```python
from build123d import *

# Parameters (mm, degrees)
SALIENTE_EXTRUIR1_DEPTH = 20
CORTAR_EXTRUIR1_START   = -6.736039
CROQUIS2_W              = 14
CROQUIS2_H              = 7.5
CORTAR_EXTRUIR1_DEPTH   = 6.736039
CORTAR_EXTRUIR2_REACH   = 29.226
CROQUIS3_R              = 1.7
CROQUIS5_W              = 14
CROQUIS5_H              = 5.763961031
CORTAR_EXTRUIR4_DEPTH   = 10
CORTAR_EXTRUIR3_REACH   = 30.507
CROQUIS4_R              = 3.75
CROQUIS4_W              = 5
CROQUIS4_H              = 5
REDONDEO1_R             = 5
REDONDEO2_R             = 5
REDONDEO3_R             = 2


# Some blends are built 0.0001 mm under size
with BuildPart() as part:
    # Croquis1 → Saliente-Extruir1 (new body)
    with BuildSketch(Plane(origin=(0, 0, 0), x_dir=(0, 0, -1), z_dir=(1, 0, 0))):
        Polygon((-3.75, 4.25), (-0.85, 4.25), (3.15, 8.25), (3.15, 16.813961031), (7.65, 16.813961031), (7.65, 6.386038969), (3.75, 2.486038969), (3.75, -4.25), (-3.75, -4.25), align=None)
    extrude(amount=SALIENTE_EXTRUIR1_DEPTH)

    # Croquis2 → Cortar-Extruir1 (cut)
    with BuildSketch(Plane.XZ.offset(4.25).offset(CORTAR_EXTRUIR1_START)):
        with Locations((10, 0)):
            Rectangle(CROQUIS2_W, CROQUIS2_H)
    extrude(amount=CORTAR_EXTRUIR1_DEPTH, mode=Mode.SUBTRACT)

    # Cortar-Extruir2: up to this face of the body (flat: up to its plane)
    cortar_extruir2_end = Plane(part.part.faces().sort_by_distance((20, 4.974035109, -2.43613322))[0])
    # Croquis3 → Cortar-Extruir2 (cut, up to the picked face)
    with BuildSketch(Plane.ZY, mode=Mode.PRIVATE) as cortar_extruir2_sk1:
        Circle(CROQUIS3_R)
    cortar_extruir2_tool1 = split(extrude(cortar_extruir2_sk1.sketch, amount=-CORTAR_EXTRUIR2_REACH, mode=Mode.PRIVATE), bisect_by=cortar_extruir2_end, keep=Keep.BOTH, mode=Mode.PRIVATE)
    add(cortar_extruir2_tool1.solids().sort_by(Axis((0, 0, 0), (1, 0, 0)))[0], mode=Mode.SUBTRACT)

    # Croquis5 → Cortar-Extruir4 (cut)
    with BuildSketch(Plane.XY.offset(-3.15)):
        with Locations((10, 5.368019484)):
            Rectangle(CROQUIS5_W, CROQUIS5_H)
    extrude(amount=CORTAR_EXTRUIR4_DEPTH, mode=Mode.SUBTRACT)

    # Cortar-Extruir3: up to this face of the body (flat: up to its plane)
    cortar_extruir3_end = Plane(part.part.faces().sort_by_distance((10, 10.237705939, -3.15))[0])
    # Croquis4 → Cortar-Extruir3 (cut, up to the picked face)
    with BuildSketch(Plane(origin=(0, 0, -7.65), x_dir=(-1, 0, 0), z_dir=(0, 0, -1)), mode=Mode.PRIVATE) as cortar_extruir3_sk1:
        with Locations((-10, 11.6)):
            Circle(CROQUIS4_R)
    cortar_extruir3_tool1 = split(extrude(cortar_extruir3_sk1.sketch, amount=-CORTAR_EXTRUIR3_REACH, mode=Mode.PRIVATE), bisect_by=cortar_extruir3_end, keep=Keep.BOTH, mode=Mode.PRIVATE)
    # Croquis4 → Cortar-Extruir3 (cut, up to the picked face)
    with BuildSketch(Plane(origin=(0, 0, -7.65), x_dir=(-1, 0, 0), z_dir=(0, 0, -1)), mode=Mode.PRIVATE) as cortar_extruir3_sk2:
        with Locations((-17.5, 14.313961031)):
            Rectangle(CROQUIS4_W, CROQUIS4_H)
    cortar_extruir3_tool2 = split(extrude(cortar_extruir3_sk2.sketch, amount=-CORTAR_EXTRUIR3_REACH, mode=Mode.PRIVATE), bisect_by=cortar_extruir3_end, keep=Keep.BOTH, mode=Mode.PRIVATE)
    # Croquis4 → Cortar-Extruir3 (cut, up to the picked face)
    with BuildSketch(Plane(origin=(0, 0, -7.65), x_dir=(-1, 0, 0), z_dir=(0, 0, -1)), mode=Mode.PRIVATE) as cortar_extruir3_sk3:
        with Locations((-2.5, 14.313961031)):
            Rectangle(CROQUIS4_W, CROQUIS4_H)
    cortar_extruir3_tool3 = split(extrude(cortar_extruir3_sk3.sketch, amount=-CORTAR_EXTRUIR3_REACH, mode=Mode.PRIVATE), bisect_by=cortar_extruir3_end, keep=Keep.BOTH, mode=Mode.PRIVATE)
    # Croquis4 → Cortar-Extruir3 (cut, up to the picked face)
    with BuildSketch(Plane(origin=(0, 0, -7.65), x_dir=(-1, 0, 0), z_dir=(0, 0, -1)), mode=Mode.PRIVATE) as cortar_extruir3_sk4:
        Polygon((-15, 6.486038969), (-5, 6.486038969), (-3, 2.486038969), (-17, 2.486038969), align=None)
    cortar_extruir3_tool4 = split(extrude(cortar_extruir3_sk4.sketch, amount=-CORTAR_EXTRUIR3_REACH, mode=Mode.PRIVATE), bisect_by=cortar_extruir3_end, keep=Keep.BOTH, mode=Mode.PRIVATE)
    add(cortar_extruir3_tool1.solids().sort_by(Axis((10, 11.6, -7.65), (0, 0, 1)))[0], mode=Mode.SUBTRACT)
    add(cortar_extruir3_tool2.solids().sort_by(Axis((17.5, 14.313961, -7.65), (0, 0, 1)))[0], mode=Mode.SUBTRACT)
    add(cortar_extruir3_tool3.solids().sort_by(Axis((2.5, 14.313961, -7.65), (0, 0, 1)))[0], mode=Mode.SUBTRACT)
    add(cortar_extruir3_tool4.solids().sort_by(Axis((10, 4.374928, -7.65), (0, 0, 1)))[0], mode=Mode.SUBTRACT)

    # Redondeo1
    redondeo1_edges = [part.edges().sort_by_distance(p)[0] for p in [
        (5, 11.813961031, -5.4),
        (15, 11.813961031, -5.4),
    ]]
    fillet(redondeo1_edges, radius=REDONDEO1_R - 0.0001)  # a hair under: the kernel refuses the full size

    # Redondeo2
    # the kernel refuses this fillet: 5 mm, written as the material it takes off along each edge
    with BuildSketch(Plane(origin=(15, 16.813961031, -16.800740757), x_dir=(-1, 0, 0), z_dir=(0, 0, 1))) as redondeo2_piece_1:
        with BuildLine():
            CenterArc((3.660296303, 5), REDONDEO2_R, 209.9996692, 60.0003308)
            Line((-0.66984515, 2.500025), (-1.102859295, 2.2500275))
            ThreePointArc((-1.102859295, 2.2500275), (-0.5, 0.0001), (-0.5, 0))
            Line((-0.5, 0), (0, -0.5))
            Line((0, -0.5), (3.660296303, -0.5))
            Line((3.660296303, -0.5), (3.660296303, 0))
        make_face()
    extrude(amount=22.801481513, mode=Mode.SUBTRACT)
    with BuildSketch(Plane(origin=(5, 16.813961031, -16.800740757), x_dir=(-0.258806597579155, -0.9659291615069406, 0), z_dir=(0, 0, 1)), Plane(origin=(20, 11.813961031, -16.800740757), x_dir=(-0.9659291615069399, 0.25880659757915725, 0), z_dir=(0, 0, 1))) as redondeo2_piece_2:
        with BuildLine():
            CenterArc((3.882336975, 4.829619926), REDONDEO2_R, 194.999261652, 60.0003308)
            Line((-0.947308832, 3.535586938), (-1.430273413, 3.40618364))
            Line((-1.430273413, 3.40618364), (-0.482964581, -0.129403299))
            Line((-0.482964581, -0.129403299), (0.129403299, -0.482964581))
            ThreePointArc((0.129403299, -0.482964581), (0.129499892, -0.4829387), (2.458794439, -0.482961993))
            Line((2.458794439, -0.482961993), (2.588207396, 0))
        make_face()
    extrude(amount=22.801481513, mode=Mode.SUBTRACT)
    with BuildSketch(Plane(origin=(0, 11.813961031, -16.800740757), x_dir=(0.9659291615069402, 0.2588065975791559, 0), z_dir=(0, 0, 1))) as redondeo2_piece_3:
        with BuildLine():
            CenterArc((3.882336975, -4.829619926), REDONDEO2_R, 105.000407548, 60.0003308)
            Line((-0.947308832, -3.535586938), (-1.430273413, -3.40618364))
            Line((-1.430273413, -3.40618364), (-0.482964581, 0.129403299))
            Line((-0.482964581, 0.129403299), (0.129403299, 0.482964581))
            ThreePointArc((0.129403299, 0.482964581), (0.129499892, 0.4829387), (2.458794439, 0.482961993))
            Line((2.458794439, 0.482961993), (2.588207396, 0))
        make_face()
    extrude(amount=22.801481513, mode=Mode.SUBTRACT)

    # Redondeo3
    redondeo3_edges = [part.edges().sort_by_distance(p)[0] for p in [
        (15, 6.486038969, -5.4),
        (5, 6.486038969, -5.4),
        (1.500464067, 8.25, -3.15),
        (18.499535933, 8.25, -3.15),
        (18.5, 4.25, 3.75),
        (1.5, 4.25, 3.75),
    ]]
    fillet(redondeo3_edges, radius=REDONDEO3_R)


solid = part.part
```
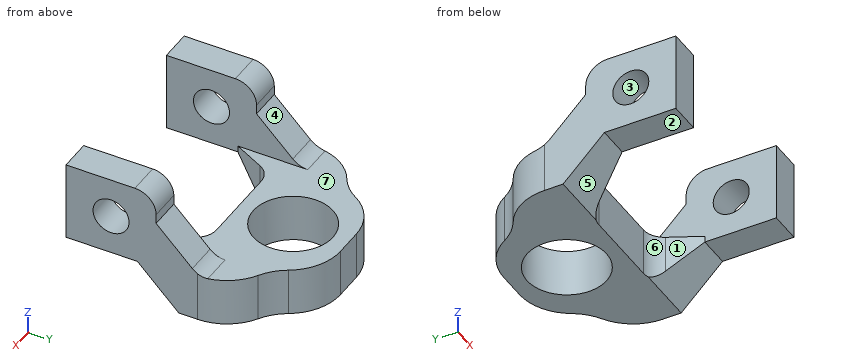
The model under review builds one solid part; all positions refer to its coordinate system, in mm. Face numbers are marked on the shaded views. A direction names the side the tool comes from. Round coordinates to 2 decimals unless told otherwise and drop trailing zeros. Loops run counter-clockwise (first coordinate to the right, second up) from the corner with the lowest first, then second, coordinate; pieces in that order, holes last.
Item 1: Take a section at A-A (z = 0). Write out the cut boundary in (x, y), then the cut area to 3 significant figures.
Determined:
outline: (0, -4.25) - (3, -4.25) - (3, -1.7) - (0, -1.7) - close; (0, 1.7) - (3, 1.7) - (3, 5.1) - (0, 5.1) - close; (17, -4.25) - (20, -4.25) - (20, -1.7) - (17, -1.7) - close; (17, 1.7) - (20, 1.7) - (20, 5.1) - (17, 5.1) - close
area: 35.7 mm2
Item 2: Take a section at C-C (y = -2.25). Write out the cut boundary in (x, z).
Determined:
outline: (0, -3.75) - (3, -3.75) - (3, 3.75) - (0, 3.75) - close; (17, -3.75) - (20, -3.75) - (20, 3.75) - (17, 3.75) - close
Item 3: Take a section at B-B (x = 10). Write out the cut boundary in (y, z).
Determined:
outline: (6.49, -7.65) - (7.85, -7.65) - (7.85, -3.15) - (6.49, -3.15) - close; (15.35, -7.65) - (16.81, -7.65) - (16.81, -3.15) - (15.35, -3.15) - close
Item 4: Clearance check with flat-ended pins moving along their axes: pin 1 Ø0.7 at (x, z) = (19, 1) entering from +Y; pin 2 Ø2.5 at (x, y) = (18.5, 0) entering from -Z; pin 3 Ø1 at (x, z) = (2, 1.5) entering from +Y. State where each tip first meets the part, or that it passes through.
Determined:
pin 1: stops at y = 4.45
pin 2: stops at z = -3.75
pin 3: stops at y = 4.25
Item 5: Mouldability with a two-part tool opening along Z and no side actions: class the marked faces 1, 2, 3 and 4 as released by +Z, released by -Z, zero draft, split by the parting line, or undercut.
Determined:
face 1: zero draft
face 2: released by -Z
face 3: undercut
face 4: released by +Z
Item 6: For line 1 (X direction, y = 1.75, z = -2.5); line 2 (Z direction, x = 14.5, y = 8.25); line 3 (Y direction, x = 10, z = -4.6), list the stretches that pass through material, from the lowest coordinate up.
Determined:
line 1: x = 0 to 3, 17 to 20
line 2: z = -7.65 to -3.15
line 3: y = 6.49 to 7.85, 15.35 to 16.81
Item 7: For the marked faces 5, 6 and 7, list the 3-axis set-ups (+Z, -Z, +X, -X, +Y, -Y) from which the entire face can be reached by the end or side of a thin tool; tool diameter is ignored.
Determined:
face 5: -Z, +X, -X, -Y
face 6: +Z, -Z, -Y
face 7: +Z, +Y
Item 8: Take a section at D-D (y = 0). Write out the cut boundary in (x, z), then the cut area to 3 significant figures.
Determined:
outline: (0, -3.75) - (3, -3.75) - (3, -1.7) - (0, -1.7) - close; (0, 1.7) - (3, 1.7) - (3, 3.75) - (0, 3.75) - close; (17, -3.75) - (20, -3.75) - (20, -1.7) - (17, -1.7) - close; (17, 1.7) - (20, 1.7) - (20, 3.75) - (17, 3.75) - close
area: 24.6 mm2
